Could you check a few things on this drawing? It's one solid part, dimensions in mm from its lowest x, y, z. Coordinates: 2 decimals unless noted, no trailing zeros. Order: outer loops, then holes, each group sorted by start corner. A loop starts at its lowest first (then second) coordinate and runs counter-clockwise, first axis right, second up. Notation, with made-up numbers: (-6, 4.5) - (5, 4.5) arc R18 cw to (5, 27.5) - close; hole circle Ø1 at (-1.75, 83). An arc over 180 degrees is marked (long way). Return JSON: item names as keys, results as strings. Group by question number.
1) Imagine slicing it at C-C (x = 4). Write out the boundary of the cut face in (y, z), and give its area (3 significant figures).
2) If I drill on line 1 along Z through (x, y) = (24, 0.85); line 2 along Z through (x, y) = (24, 2.25), over which ranges is the centre line in solid material (lowest first)?
3) For pin 1 Ø10 at (x, z) = (13.5, 15.5) entering from +Y; pin 2 Ø1.5 at (x, z) = (24, 4) entering from -Y, each with a flat end and sliding along its axis, tell me the tip position at first contact or that it passes through.
4) Imagine slicing it at A-A (y = 1.4). Write out the boundary of the cut face in (x, z).
5) Imagine slicing it at B-B (z = 4). Write out the boundary of the cut face in (x, y), and give its area (3 significant figures).
6) If we mould it in two halves opening along X, with no side actions, what happens to the marked faces 1 and 2? For each: pulls with the +X half, pulls with the -X half, needs draft (parallel to the pull), parting line crosses it, or undercut.
7) Imagine slicing it at D-D (x = 12.5). Write out the boundary of the cut face in (y, z), and give its area (3 significant figures).
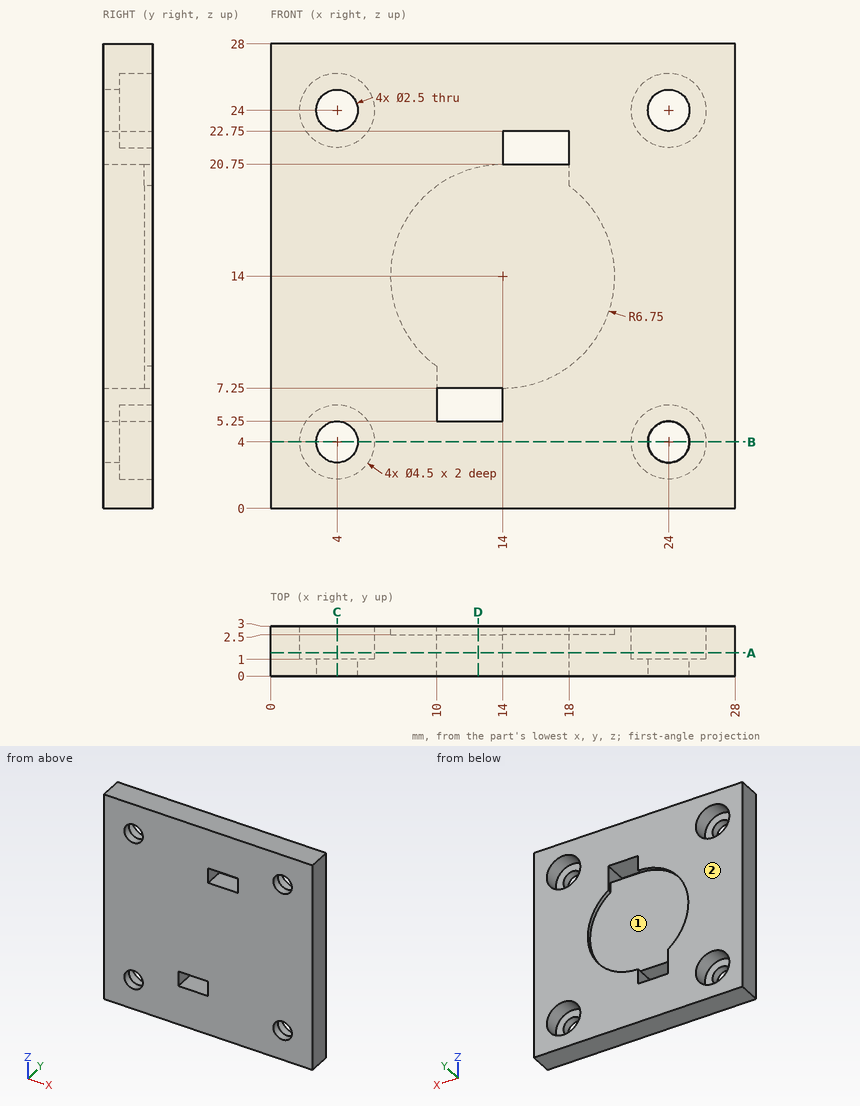
Calculated:
{
 "1": {"outline": "(0, 0) - (3, 0) - (3, 1.75) - (1, 1.75) - (1, 2.75) - (0, 2.75) - close; (0, 5.25) - (1, 5.25) - (1, 6.25) - (3, 6.25) - (3, 21.75) - (1, 21.75) - (1, 22.75) - (0, 22.75) - close; (0, 25.25) - (1, 25.25) - (1, 26.25) - (3, 26.25) - (3, 28) - (0, 28) - close", "area": "61.0 mm2"},
 "2": {"line 1": "0 to 2.75, 5.25 to 22.75, 25.25 to 28", "line 2": "0 to 1.75, 6.25 to 21.75, 26.25 to 28"},
 "3": {"pin 1": "y = 2.5", "pin 2": "through"},
 "4": {"outline": "(0, 0) - (28, 0) - (28, 28) - (0, 28) - close; hole circle Ø4.5 at (4, 4); hole circle Ø4.5 at (4, 24); hole (10, 5.25) - (14, 5.25) - (14, 7.25) - (10, 7.25) - close; hole (14, 20.75) - (18, 20.75) - (18, 22.75) - (14, 22.75) - close; hole circle Ø4.5 at (24, 4); hole circle Ø4.5 at (24, 24)"},
 "5": {"outline": "(0, 0) - (2.75, 0) - (2.75, 1) - (1.75, 1) - (1.75, 3) - (0, 3) - close; (5.25, 0) - (22.75, 0) - (22.75, 1) - (21.75, 1) - (21.75, 3) - (6.25, 3) - (6.25, 1) - (5.25, 1) - close; (25.25, 0) - (28, 0) - (28, 3) - (26.25, 3) - (26.25, 1) - (25.25, 1) - close", "area": "61.0 mm2"},
 "6": {"face 1": "undercut", "face 2": "needs draft"},
 "7": {"outline": "(0, 0) - (3, 0) - (3, 5.25) - (0, 5.25) - close; (0, 7.25) - (2.5, 7.25) - (2.5, 20.58) - (3, 20.58) - (3, 28) - (0, 28) - close", "area": "71.3 mm2"}
}
